Autodesk Inventor part; units mm, degrees
ref_plane "YZ Plane" through (0, 0, 0) normal (1, 0, 0) x (0, 1, 0)
ref_plane "XZ Plane" through (0, 0, 0) normal (0, 1, 0) x (-1, 0, 0)
ref_plane "XY Plane" through (0, 0, 0) normal (0, 0, 1) x (1, 0, 0)
sketch "Sketch1" plane through (0, 0, 0) normal (0, 1, 0) x (-1, 0, 0)
  line L0 (0, 0) -> (50.8, 0)
  line L1 (50.8, 0) -> (50.8, -25.4)
  line L2 (50.8, -25.4) -> (0, -25.4)
  line L3 (0, -25.4) -> (0, 0)
  line L4 (2.54, -22.86) -> (48.26, -22.86)
  line L5 (48.26, -22.86) -> (48.26, -2.54)
  line L6 (48.26, -2.54) -> (2.54, -2.54)
  line L7 (2.54, -2.54) -> (2.54, -22.86)
  dimension "d0" = 50.8
  dimension "d1" = 25.4
  dimension "d2" = 2.54
extrude "Extrusion1" add sketch "Sketch1" against normal blind 393.7
sketch "Sketch2" plane through (-50.8, 0, 0) normal (0, 0, 1) x (1, 0, 0)
  circle A0 centre (25.4, -32.7323) radius 7.3323
  line L0 (50.8, -279.4) -> (0, -279.4)
  line L1 (50.8, -279.4) -> (50.8, 0)
  line L2 (0, 0) -> (50.8, 0)
  line L3 (0, -279.4) -> (0, 0)
  circle A1 centre (25.4, -32.7323) radius 7.3323
extrude "Extrusion2" cut sketch "Sketch2" against normal through all contours A0
properties part number "Aluminum channel pivot mount"
Work out the finished part from the listing and answer in its coordinate system (mm). A direction names the side the tool comes from. Give positions to 0.01 mm unless a question says otherwise; leave off trailing zeros. Write each loop counter-clockwise with the first axis right and the second up, starting at its lowest first coordinate (ties: lowest second). Pieces come first, ordered by that corner, then holes. Notation, with made-up numbers: (-26.75, -4) -> (26.25, -4) arc R11 cw to (26.25, 13) -> close; hole circle Ø7 at (60.25, 43). An arc over 180 degrees is marked (long way). Write each question's results on one line, items separated by ' | '.
1. Find section C-C on y = -323. Determine the outline of the cut face in (x, z), and give its area (3 significant figures).
Data:
outline: (-50.8, -25.4) -> (0, -25.4) -> (0, 0) -> (-50.8, 0) -> close; hole (-48.26, -22.86) -> (-2.54, -22.86) -> (-2.54, -2.54) -> (-48.26, -2.54) -> close | area: 361 mm^2
2. Determine the mould class of faces 1 (the flat face through (-2.54, -194, -13)), 2 (the flat face through (-25, -194, 0)), 3 (the flat face through (0, -194, -13)), 4 (the flat face through (-48.26, -194, -13)) for opening direction X: +X half, -X half, draft (parallel to the pull), parting line (faces both ways), or undercut.
Data:
face 1: undercut | face 2: draft | face 3: +X half | face 4: undercut
3. Find section B-B on z = -8. Determine the outline of the cut face in (x, y).
Data:
outline: (-50.8, -393.7) -> (-48.26, -393.7) -> (-48.26, 0) -> (-50.8, 0) -> close; (-2.54, -393.7) -> (0, -393.7) -> (0, 0) -> (-2.54, 0) -> close
4. A tool of negligible diameter and unlimited length cuts with its end or side. For faces 5 (the flat face through (-50.8, -194, -13)), 6 (the flat face through (-26, -194, -2.54)), from which of +Z, -Z, +X, -X, +Y, -Y can it reach the whole face along a straight path? Write none if from no direction.
Data:
face 5: +Z, -Z, -X, +Y, -Y | face 6: +Y, -Y
5. Straight lines are drawn through the part: L1, parallel to Z at x = -41, y = -54.5; L2, parallel to X at y = -187.5, z = -16; L3, parallel to Y at x = -25.4, z = -0.85. For each, find the intervals that lie inside material, in ascending order.
Data:
L1: -25.4 to -22.86, -2.54 to 0 | L2: -50.8 to -48.26, -2.54 to 0 | L3: -393.7 to -40.06, -25.4 to 0
6. Find section A-A on x = -25.4. Determine the outline of the cut face in (y, z).
Data:
outline: (-393.7, -25.4) -> (-40.06, -25.4) -> (-40.06, -22.86) -> (-393.7, -22.86) -> close; (-393.7, -2.54) -> (-40.06, -2.54) -> (-40.06, 0) -> (-393.7, 0) -> close; (-25.4, -25.4) -> (0, -25.4) -> (0, -22.86) -> (-25.4, -22.86) -> close; (-25.4, -2.54) -> (0, -2.54) -> (0, 0) -> (-25.4, 0) -> close
